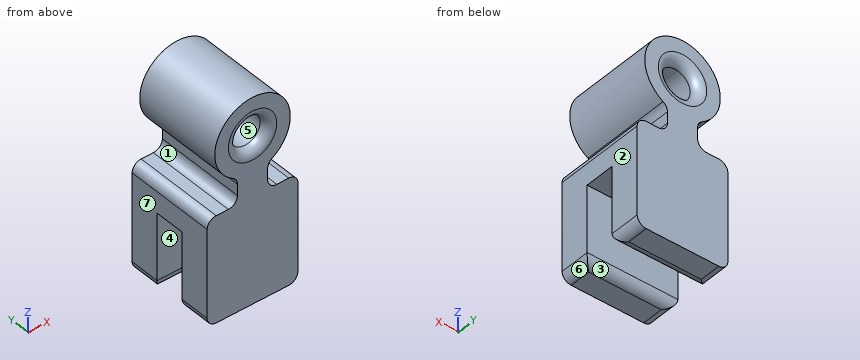
```python
from build123d import *

# Parameters (mm, degrees)
F0_R     = 5
F1_DEPTH = 30
F2_W     = 10
F2_H     = 25
F3_DEPTH = 30.001
F4_R     = 3


with BuildPart() as f1:
    # F0 (on Front) → F1 (new body)
    with BuildSketch(Plane.XZ):
        Polygon((0, 35), (0, 0), (30, 0), (30, 35), (20, 35), (10, 35), align=None)
        with BuildLine():
            Line((10, 43.5435607626), (10, 35))
            Line((10, 35), (20, 35))
            Line((20, 35), (20, 43.5435607626))
            ThreePointArc((20, 43.5435607626), (15, 67.5), (10, 43.5435607626))
        make_face()
        with Locations((15, 55)):
            Circle(F0_R, mode=Mode.SUBTRACT)
    extrude(amount=F1_DEPTH)

    # F2 (on face) → F3 (cut, through all)
    with BuildSketch(Plane.YZ.offset(30)):
        with Locations((-15, 12.5)):
            Rectangle(F2_W, F2_H)
    extrude(amount=-F3_DEPTH, mode=Mode.SUBTRACT)

    # F4
    f4_edges = [f1.edges().sort_by_distance(p)[0] for p in [
        (10, -30, 55),
        (10, 0, 55),
        (20, -15, 43.543561),
        (20, -15, 35),
        (10, -15, 35),
        (10, -15, 43.543561),
        (30, -15, 35),
        (0, -15, 35),
        (30, -25, 0),
        (30, -5, 0),
        (0, -25, 0),
        (0, -5, 0),
        (15, -20, 0),
        (15, -10, 0),
    ]]
    fillet(f4_edges, radius=F4_R)


solid = f1.part
```
Here's how the part is built. I have some questions about the finished solid (model axes, mm). Face numbers are marked on the shaded views. A direction names the side the tool comes from. Give positions to 0.01 mm unless a question says otherwise; leave off trailing zeros. Write each loop counter-clockwise with the first axis right and the second up, starting at its lowest first coordinate (ties: lowest second). Pieces come first, ordered by that corner, then holes.
(1) Thinking about a two-plate mould opening in X: for the marked faces 4, 5, 6 and 7, which applies, pulls with the +X half, pulls with the -X half, needs draft (parallel to the pull), parting line crosses it, or undercut?
Output values:
face 4: needs draft
face 5: undercut
face 6: pulls with the +X half
face 7: pulls with the -X half
(2) Imagine slicing it at D-D, the plane z = 7. Write out the boundary of the cut face in (x, y), and give its area (3 significant figures).
Output values:
outline: (0, -30) - (30, -30) - (30, -20) - (0, -20) - close; (0, -10) - (30, -10) - (30, 0) - (0, 0) - close
area: 600 mm2
(3) Imagine slicing it at C-C, the plane z = 55. Write out the boundary of the cut face in (x, y).
Output values:
outline: (2.5, -30) - (7, -30) arc R3 ccw to (10, -27) - (10, -3) arc R3 ccw to (7, 0) - (2.5, 0) - close; (20, -27) arc R3 ccw to (23, -30) - (27.5, -30) - (27.5, 0) - (23, 0) arc R3 ccw to (20, -3) - close
(4) Imagine slicing it at A-A, the plane x = 15. Write out the boundary of the cut face in (y, z).
Output values:
outline: (-30, 0) - (-23, 0) arc R3 ccw to (-20, 3) - (-20, 25) - (-10, 25) - (-10, 3) arc R3 ccw to (-7, 0) - (0, 0) - (0, 47) arc R3 ccw to (-3, 50) - (-27, 50) arc R3 ccw to (-30, 47) - close; (-30, 63) arc R3 ccw to (-27, 60) - (-3, 60) arc R3 ccw to (0, 63) - (0, 67.5) - (-30, 67.5) - close
(5) If I drill on L1, parallel to Z at x = 15, y = -10.25; L2, parallel to Y at x = 23, z = 3.5; L3, parallel to Z at x = 5, y = -18.75, over which ranges is the centre line in solid material (lowest first)?
Output values:
L1: z = 25 to 50, 60 to 67.5
L2: y = -30 to -20, -10 to 0
L3: z = 25 to 35, 47.5 to 62.5
(6) Will these pins go through, and if not, where does the flat tip stop? pin 1 (11 mm diameter, centred on x = 8.5, y = -14, fed in from -Z); pin 2 (1.5 mm diameter, centred on x = 10, y = -24.5, fed in from +Z); pin 3 (1.9 mm diameter, centred on y = -17.5, z = 40, fed in from -X).
Output values:
pin 1: stops at z = 0.4
pin 2: stops at z = 66.76
pin 3: stops at x = 10
(7) On a 3-axis mill with a long thin cutter (end or side, diameter ignored), from which of +Z, -Z, +X, -X, +Y, -Y can I reach the whole of each face in a straight line? I mean the marked faces 1, 2 and 3. Say none if no direction works.
Output values:
face 1: -X, +Y, -Y
face 2: +Z, -Z, +X, +Y, -Y
face 3: -Z, +X, -X
(8) Imagine slicing it at B-B, the plane y = -26. Write out the boundary of the cut face in (x, z), and give its area (3 significant figures).
Output values:
outline: (0, 3) arc R3 ccw to (3, 0) - (27, 0) arc R3 ccw to (30, 3) - (30, 32) arc R3 ccw to (27, 35) - (23, 35) arc R3 cw to (20, 38) - (20, 41.72) arc R3 cw to (21.45, 44.29) arc R12.5 ccw (long way) to (8.55, 44.29) arc R3 cw to (10, 41.72) - (10, 38) arc R3 cw to (7, 35) - (3, 35) arc R3 ccw to (0, 32) - close; hole circle Ø10 at (15, 55)
area: 1,540 mm2
